Could you check a few things on this model? Use its own coordinates, in mm. A direction names the side the tool comes from. Round coordinates to 2 decimals unless told otherwise and drop trailing zeros. Order: outer loops, then holes, each group sorted by start corner. A loop starts at its lowest first (then second) coordinate and runs counter-clockwise, first axis right, second up. Notation, with made-up numbers: (55, 73) - (81, 73) arc R11 cw to (81, 93) - close; hole circle Ø8 at (41.5, 59). An arc over 180 degrees is marked (long way). Use one line per item in the form item = value.
from build123d import *

# Parameters (mm, degrees)
BOSS_EXTRU_1_DEPTH                = 19
BOSS_EXTRU_1_DEPTH_BACK           = 22
ESQUISSE1_R                       = 4.9
DIAM_TRE_DU_PER_AGE_6_0_6_1_D     = 6
DIAM_TRE_DU_PER_AGE_6_0_6_1_DEPTH = 10
DIAM_TRE_DU_PER_AGE_6_0_6_1_TIP   = 1.802581857
ENL_V_MAT_EXTRU_1_REACH           = 52.813
ESQUISSE6_R                       = 1.6
DIAM_TRE_DU_PER_AGE_3_0_3_1_D     = 3
DIAM_TRE_DU_PER_AGE_3_0_3_1_DEPTH = 10
DIAM_TRE_DU_PER_AGE_3_0_3_1_TIP   = 0.901290929
TROU_TARAUD_M31_D                 = 2.5
TROU_TARAUD_M31_DEPTH             = 8.5
TROU_TARAUD_M31_TIP               = 0.751075774
CONG_1_R                          = 2
TROU_TARAUD_M32_REACH             = 59.105
TROU_TARAUD_M32_BORE_R            = 1.25
TROU_TARAUD_M41_REACH             = 59.105
TROU_TARAUD_M41_BORE_R            = 1.65
CHANFREIN1_SIZE                   = 0.2
TROU_TARAUD_M33_D                 = 2.5


with BuildPart() as part:
    # Esquisse1 → Boss.-Extru.1 (new, two sides: drawn at the far end of the back side and taken through both)
    with BuildSketch(Plane.XY.offset(-BOSS_EXTRU_1_DEPTH_BACK)):
        Polygon((-4, -7), (-4, -37), (-14, -37), (-14, -7), (-29, -7), (-29, 7), (-14, 7), (-14, 37), (-4, 37), (-4, 7), (23, 7), (23, -7), align=None)
        Circle(ESQUISSE1_R, mode=Mode.SUBTRACT)
    extrude(amount=BOSS_EXTRU_1_DEPTH + BOSS_EXTRU_1_DEPTH_BACK)

    # Diamètre du perçage Ø6.0 (6)1
    with Locations(Plane(origin=(23, 0, 0), x_dir=(0, 0, -1), z_dir=(1, 0, 0))):
        with Locations((0, 0)):
            Hole(DIAM_TRE_DU_PER_AGE_6_0_6_1_D / 2, depth=DIAM_TRE_DU_PER_AGE_6_0_6_1_DEPTH)
            with Locations((0, 0, -(DIAM_TRE_DU_PER_AGE_6_0_6_1_DEPTH + DIAM_TRE_DU_PER_AGE_6_0_6_1_TIP / 2))):  # 118° drill point
                Cone(0, DIAM_TRE_DU_PER_AGE_6_0_6_1_D / 2, DIAM_TRE_DU_PER_AGE_6_0_6_1_TIP, mode=Mode.SUBTRACT)

    # Esquisse6 → Enlèv. mat.-Extru.1 (cut, up to next)
    with BuildSketch(Plane(origin=(-4, 0, 0), x_dir=(0, 0, -1), z_dir=(1, 0, 0)), mode=Mode.PRIVATE) as enl_v_mat_extru_1_sk1:
        with Locations(Location((18, -11, 0), (0, 0, 90))):
            Circle(ESQUISSE6_R)
    enl_v_mat_extru_1_tool1 = extrude(enl_v_mat_extru_1_sk1.sketch, amount=-ENL_V_MAT_EXTRU_1_REACH, mode=Mode.PRIVATE) & part.part
    # Esquisse6 → Enlèv. mat.-Extru.1 (cut, up to next)
    with BuildSketch(Plane(origin=(-4, 0, 0), x_dir=(0, 0, -1), z_dir=(1, 0, 0)), mode=Mode.PRIVATE) as enl_v_mat_extru_1_sk2:
        with Locations(Location((-4, -33, 0), (0, 0, 90))):
            Circle(ESQUISSE6_R)
    enl_v_mat_extru_1_tool2 = extrude(enl_v_mat_extru_1_sk2.sketch, amount=-ENL_V_MAT_EXTRU_1_REACH, mode=Mode.PRIVATE) & part.part
    add(enl_v_mat_extru_1_tool1.solids().sort_by_distance((-4, -11, -18))[0], mode=Mode.SUBTRACT)
    add(enl_v_mat_extru_1_tool2.solids().sort_by_distance((-4, -33, 4))[0], mode=Mode.SUBTRACT)

    # Diamètre du perçage Ø3.0 (3)1
    with Locations(Plane.ZY.offset(29)):
        with Locations((0, 0)):
            Hole(DIAM_TRE_DU_PER_AGE_3_0_3_1_D / 2, depth=DIAM_TRE_DU_PER_AGE_3_0_3_1_DEPTH)
            with Locations((0, 0, -(DIAM_TRE_DU_PER_AGE_3_0_3_1_DEPTH + DIAM_TRE_DU_PER_AGE_3_0_3_1_TIP / 2))):  # 118° drill point
                Cone(0, DIAM_TRE_DU_PER_AGE_3_0_3_1_D / 2, DIAM_TRE_DU_PER_AGE_3_0_3_1_TIP, mode=Mode.SUBTRACT)

    # Trou taraudé M31
    with Locations(Plane.XY.offset(19)):
        with Locations((-9, 32), (-9, -32)):
            Hole(TROU_TARAUD_M31_D / 2, depth=TROU_TARAUD_M31_DEPTH)
            with Locations((0, 0, -(TROU_TARAUD_M31_DEPTH + TROU_TARAUD_M31_TIP / 2))):  # 118° drill point
                Cone(0, TROU_TARAUD_M31_D / 2, TROU_TARAUD_M31_TIP, mode=Mode.SUBTRACT)

    # Congé1
    cong_1_edges = [part.edges().sort_by_distance(p)[0] for p in [
        (-29, 0, -22),
        (-9, -37, -22),
        (23, 0, -22),
        (-9, 37, -22),
    ]]
    fillet(cong_1_edges, radius=CONG_1_R)

    # Trou taraudé M32 bore → Trou taraudé M32 (cut, up to next)
    with BuildSketch(Plane(origin=(0, -7, 0), x_dir=(-1, 0, 0), z_dir=(0, -1, 0)), mode=Mode.PRIVATE) as trou_taraud_m32_sk1:
        with Locations((25, 0)):
            Circle(TROU_TARAUD_M32_BORE_R)
    trou_taraud_m32_tool1 = extrude(trou_taraud_m32_sk1.sketch, amount=-TROU_TARAUD_M32_REACH, mode=Mode.PRIVATE) & part.part
    # Trou taraudé M32 bore → Trou taraudé M32 (cut, up to next)
    with BuildSketch(Plane(origin=(0, -7, 0), x_dir=(-1, 0, 0), z_dir=(0, -1, 0)), mode=Mode.PRIVATE) as trou_taraud_m32_sk2:
        with Locations((0, -11)):
            Circle(TROU_TARAUD_M32_BORE_R)
    trou_taraud_m32_tool2 = extrude(trou_taraud_m32_sk2.sketch, amount=-TROU_TARAUD_M32_REACH, mode=Mode.PRIVATE) & part.part
    add(trou_taraud_m32_tool1.solids().sort_by_distance((-25, -7, 0))[0], mode=Mode.SUBTRACT)
    add(trou_taraud_m32_tool2.solids().sort_by_distance((0, -7, 11))[0], mode=Mode.SUBTRACT)

    # Trou taraudé M41 bore → Trou taraudé M41 (cut, up to next)
    with BuildSketch(Plane(origin=(0, -7, 0), x_dir=(-1, 0, 0), z_dir=(0, -1, 0)), mode=Mode.PRIVATE) as trou_taraud_m41_sk1:
        with Locations((-18, 0)):
            Circle(TROU_TARAUD_M41_BORE_R)
    trou_taraud_m41_tool1 = extrude(trou_taraud_m41_sk1.sketch, amount=-TROU_TARAUD_M41_REACH, mode=Mode.PRIVATE) & part.part
    add(trou_taraud_m41_tool1.solids().sort_by_distance((18, -7, 0))[0], mode=Mode.SUBTRACT)

    # Chanfrein1
    chanfrein1_edges = [part.edges().sort_by_distance(p)[0] for p in [
        (-4.9, 0, -22),
        (23, 0, -3),
        (-29, 0, 1.5),
    ]]
    chamfer(chanfrein1_edges, length=CHANFREIN1_SIZE)

    # Trou taraudé M33 (through all)
    with Locations(Plane(origin=(-4, 0, 0), x_dir=(0, 0, -1), z_dir=(1, 0, 0))):
        with Locations((18, 33), (-4, 11)):
            Hole(TROU_TARAUD_M33_D / 2)


solid = part.part
Item 1: Imagine slicing it at B-B on y = -11. Please give me the cut outline in (x, z).
Found:
outline = (-14, -22) - (-4, -22) - (-4, -19.6) - (-14, -19.6) - close; (-14, -16.4) - (-4, -16.4) - (-4, 19) - (-14, 19) - close
Item 2: Imagine slicing it at C-C on x = 18. Please give me the cut outline in (y, z), plus the area to 3 significant figures.
Found:
outline = (-7, -22) - (7, -22) - (7, 19) - (-7, 19) - (-7, 1.65) - (-2.51, 1.65) arc R3 cw (long way) to (-2.51, -1.65) - (-7, -1.65) - close
area = 532 mm2
Item 3: Will these pins go through, and if not, where does the flat tip stop? P1, Ø4, axis at x = 2, y = 2, coming from the -Z side; P2, Ø15, axis at y = 16.5, z = -10, coming from the -X side; P3, Ø2, axis at x = -16.5, z = -2, coming from the -Y side; P4, Ø4.5, axis at x = 18, z = 0, coming from the +Y side.
Found:
P1 = through
P2 = -14
P3 = -7
P4 = 7
Item 4: For faces 4 (the face through (-21, -7, -2)), 5 (the face through (-4, -22, -2)), 6 (the face through (-1.19, -5.88, 10.62)), which set-ups out of +Z, -Z, +X, -X, +Y, -Y let a thin tool reach every point of the face, with its end or its side?
Found:
face_4 = +Z, -Z, -X, -Y
face_5 = +Z, -Z, +X, -Y
face_6 = -Y
Item 5: If we mould it in two halves opening along Y, with no side actions, what happens to faces 1 (the face through (-26.155, -3.958, 0.479)), 2 (the face through (-8.93, 36.4, -21.43)), 3 (the face through (-9.028, 32.215, 9.879))? For each: released by +Y, released by -Y, zero draft, split by the parting line, or undercut.
Found:
face_1 = zero draft
face_2 = released by +Y
face_3 = undercut
Item 6: Imagine slicing it at A-A on z = -12.5. Please give me the cut outline in (x, y), plus the area to 3 significant figures.
Found:
outline = (-29, -7) - (-14, -7) - (-14, -37) - (-4, -37) - (-4, -7) - (23, -7) - (23, 7) - (-4, 7) - (-4, 37) - (-14, 37) - (-14, 7) - (-29, 7) - close; hole circle Ø9.8 at (0, 0)
area = 1,250 mm2
Item 7: I need wall thicknesses on L1, parallel to X at y = 32, z = 13.5; L2, parallel to Y at x = 7, z = -14.5; L3, parallel to Z at x = 18, y = -4.85. Which ranges of each line are inside material? Lowest first, please.
Found:
L1 = -14 to -10.25, -7.75 to -4
L2 = -7 to 7
L3 = -22 to -1.65, 1.65 to 19
Item 8: Imagine slicing it at D-D on z = 16.5. Please give me the cut outline in (x, y).
Found:
outline = (-29, -7) - (-14, -7) - (-14, -37) - (-4, -37) - (-4, -7) - (23, -7) - (23, 7) - (-4, 7) - (-4, 37) - (-14, 37) - (-14, 7) - (-29, 7) - close; hole circle Ø2.5 at (-9, -32); hole circle Ø2.5 at (-9, 32); hole circle Ø9.8 at (0, 0)
